```python
from build123d import *

# Parameters (mm, degrees)
F0_W     = 5.842
F0_H     = 12.7
F0_R     = 3.175
F2_DEPTH = 3.175
F3_R     = 1.524
F4_DEPTH = 6.35


with BuildPart() as f1:
    # F0 (on Front) → F1 (revolve)
    with BuildSketch(Plane.XZ):
        Polygon((5.842, 12.7), (5.842, 0), (66.294, 0), (66.294, 12.7), (56.134, 12.7), (56.134, 10.16), (10.16, 10.16), (10.16, 12.7), align=None)
        with Locations((2.921, 6.35)):
            Rectangle(F0_W, F0_H)
    revolve(axis=Axis((33.147, 0, 0), (-1, 0, 0)))

    # F0 (on Front) → F2 (join, symmetric)
    with BuildSketch(Plane.XZ):
        with BuildLine():
            Line((-0.9398, 0), (0, 0))
            Line((0, 0), (0, 12.7))
            Line((0, 12.7), (5.842, 12.7))
            Line((5.842, 12.7), (5.842, 15.24))
            Line((5.842, 15.24), (-0.508, 15.24))
            Line((-0.508, 15.24), (-10.8806298187, 3.8475430269))
            ThreePointArc((-10.8806298187, 3.8475430269), (-4.5919612295, 5.3297205562), (-0.9398, 0))
        make_face()
        with Locations((2.921, 6.35)):
            Rectangle(F0_W, F0_H)
        with BuildLine():
            Line((5.842, 0), (0, 0))
            Line((0, 0), (-0.9398, 0))
            ThreePointArc((-0.9398, 0), (-3.1957909266, -4.5493385486), (-8.1826630726, -5.5069827884))
            Line((-8.1826630726, -5.5069827884), (5.842, -9.398))
            Line((5.842, -9.398), (5.842, 0))
        make_face()
        with BuildLine():
            ThreePointArc((-8.1826630726, -5.5069827884), (-3.1957909266, -4.5493385486), (-0.9398, 0))
            ThreePointArc((-0.9398, 0), (-4.5919612295, 5.3297205562), (-10.8806298187, 3.8475430269))
            ThreePointArc((-10.8806298187, 3.8475430269), (-12.1459778134, -1.5837270034), (-8.1826630726, -5.5069827884))
        make_face()
        with Locations((-6.6548, 0)):
            Circle(F0_R, mode=Mode.SUBTRACT)
    extrude(amount=F2_DEPTH, both=True)

    # F3 (on face) → F4 (join, symmetric)
    with BuildSketch(Plane.YZ.offset(66.294)):
        with BuildLine():
            ThreePointArc((-5.08, 0), (0, 5.08), (5.08, 0))
            Line((5.08, 0), (5.08, 11.6397422652))
            ThreePointArc((5.08, 11.6397422652), (0, 12.7), (-5.08, 11.6397422652))
            Line((-5.08, 11.6397422652), (-5.08, 0))
        make_face()
        with BuildLine():
            ThreePointArc((-5.08, 0), (0, -5.08), (5.08, 0))
            ThreePointArc((5.08, 0), (0, 5.08), (-5.08, 0))
        make_face()
        Circle(F3_R, mode=Mode.SUBTRACT)
        with BuildLine():
            ThreePointArc((-5.08, 11.6397422652), (0, 12.7), (5.08, 11.6397422652))
            Line((5.08, 11.6397422652), (5.08, 15.24))
            Line((5.08, 15.24), (-5.08, 15.24))
            Line((-5.08, 15.24), (-5.08, 11.6397422652))
        make_face()
    extrude(amount=F4_DEPTH, both=True)


solid = f1.part
```
Geometry: final body of the model. Coordinates: model frame, mm. A direction names the side the tool comes from. Coordinates: 2 decimals unless noted, no trailing zeros. Order: outer loops, then holes, each group sorted by start corner. A loop starts at its lowest first (then second) coordinate and runs counter-clockwise, first axis right, second up. Notation, with made-up numbers: M 60,42 L 80,42 A10 ccw 80,61 Z; hole C 5.5,-28 d4. An arc over 180 degrees is marked long. Answer as CSV lines item,"result".
Q1. Line query: probe 1 along Y at (x, z) = (69, 0); probe 2 along Z at (x, y) = (69.25, 0); probe 3 along X at (y, z) = (10.25, 4.5). Output: solid intervals per line, ascending. Write a range as [from, to].
Answers:
probe 1,"y = [-5.08, -1.52], [1.52, 5.08]"
probe 2,"z = [-5.08, -1.52], [1.52, 15.24]"
probe 3,"x = [0, 10.16], [56.13, 66.29]"
Q2. Section D-D on z = -4.25. Return the cut outline in (x, y) (3 decimals), and give its area (3 significant figures).
Answers:
outline,"M -10.476,-3.175 L 0,-3.175 L 0,-11.968 L 10.16,-11.968 L 10.16,-9.228 L 56.134,-9.228 L 56.134,-11.968 L 66.294,-11.968 L 66.294,-2.783 L 72.644,-2.783 L 72.644,2.783 L 66.294,2.783 L 66.294,11.968 L 56.134,11.968 L 56.134,9.228 L 10.16,9.228 L 10.16,11.968 L 0,11.968 L 0,3.175 L -10.476,3.175 Z"
area,"1,440 mm^2"
Q3. Section C-C on y = 8.5. Return the cut outline in (x, z), and give its area (3 significant figures).
Answers:
outline,"M 0,-9.44 L 10.16,-9.44 L 10.16,-5.57 L 56.13,-5.57 L 56.13,-9.44 L 66.29,-9.44 L 66.29,9.44 L 56.13,9.44 L 56.13,5.57 L 10.16,5.57 L 10.16,9.44 L 0,9.44 Z"
area,"895 mm^2"
Q4. First-contact query: P1, Ø4, axis at x = 52, y = -3.5, coming from the -Z side; P2, Ø5.5, axis at x = 0, z = 6.5, coming from the -Y side; P3, Ø6, axis at x = -1.5, y = 8, coming from the -Z side. Flat tips, straight axial feed; report the tip coordinate or a pass-through.
Answers:
P1,"stops at z = -10.05"
P2,"stops at y = -12.13"
P3,"stops at z = -11.49"
Q5. Draft query along Z for faces 6 (the cylindrical face through (69.42, -0.2, 1.51)), 7 (the flat face through (-5.622, -0.044, 9.624)), 8 (the flat face through (-3, -3.175, 4)). Return one class per face: pulls with the +Z half, pulls with the -Z half, needs draft (parallel to the pull), parting line crosses it, or undercut.
Answers:
face 6,"undercut"
face 7,"pulls with the +Z half"
face 8,"needs draft"
Q6. Set-up query: faces 1 (the flat face through (72.644, 0, 5)), 2 (the flat face through (68, 5.08, 9)), 3 (the flat face through (68, -5.08, 9)), 4 (the flat face through (0, -5, 0)), 5 (the cylindrical face through (32.825, 10.074, -1.323)). Return all of +Z, -Z, +X, -X, +Y, -Y with unobstructed straight access to the full face (end or side cutting, diameter ignored); none if empty.
Answers:
face 1,"+Z, -Z, +X, +Y, -Y"
face 2,"+Z, +X, +Y"
face 3,"+Z, +X, -Y"
face 4,"-Z, -X"
face 5,"none"
Q7. Section A-A on y = 0. Return the cut outline in (x, z) (3 decimals), and give its area (3 significant figures).
Answers:
outline,"M -10.881,3.848 A5.715 ccw -8.183,-5.507 L 0,-7.777 L 0,-12.7 L 10.16,-12.7 L 10.16,-10.16 L 56.134,-10.16 L 56.134,-12.7 L 66.294,-12.7 L 66.294,-5.08 L 72.644,-5.08 L 72.644,-1.524 L 66.294,-1.524 L 66.294,1.524 L 72.644,1.524 L 72.644,15.24 L 59.944,15.24 L 59.944,12.7 L 56.134,12.7 L 56.134,10.16 L 10.16,10.16 L 10.16,12.7 L 5.842,12.7 L 5.842,15.24 L -0.508,15.24 Z; hole C -6.655,0 d6.35"
area,"1,740 mm^2"
Q8. Section B-B on x = -6. Return the cut outline in (y, z) (3 decimals).
Answers:
outline,"M -3.175,-6.113 L 3.175,-6.113 L 3.175,-3.107 L -3.175,-3.107 Z; M -3.175,3.107 L 3.175,3.107 L 3.175,9.208 L -3.175,9.208 Z"
